```python
from build123d import *

# Parameters (mm, degrees)
SKETCH1_W                     = 46.5
SKETCH1_H                     = 83
BOSS_EXTRUDE1_DEPTH           = 7.540625
CUT_EXTRUDE3_START            = 7.540625
CUT_EXTRUDE3_DEPTH            = 2.38125
SKETCH10_R                    = 1.35255
CUT_EXTRUDE6_DEPTH            = 4.76885
SKETCH12_R                    = 3.175
BOSS_EXTRUDE2_DEPTH           = 5.159375
BOSS_EXTRUDE2_DRAFT           = 1
BOSS_EXTRUDE2_PROFILE_2_DEPTH = 5.159375
BOSS_EXTRUDE2_PROFILE_2_DRAFT = 1
BOSS_EXTRUDE2_PROFILE_3_DEPTH = 5.159375
BOSS_EXTRUDE2_PROFILE_3_DRAFT = 1
SKETCH12_R_2                  = 2.38125
BOSS_EXTRUDE2_PROFILE_4_DEPTH = 5.159375
BOSS_EXTRUDE2_PROFILE_4_DRAFT = 1
FILLET1_R                     = 3.175


with BuildPart() as part:
    # Sketch1 → Boss-Extrude1 (new body)
    with BuildSketch(Plane(origin=(0, 0, 0), x_dir=(1, 0, 0), z_dir=(0, 1, 0))):
        Rectangle(SKETCH1_W, SKETCH1_H)
    extrude(amount=BOSS_EXTRUDE1_DEPTH)

    # Sketch2 → Cut-Extrude3 (cut)
    with BuildSketch(Plane(origin=(0, 0, 0), x_dir=(1, 0, 0), z_dir=(0, 1, 0)).offset(CUT_EXTRUDE3_START)):
        with BuildLine():
            Line((5.926342072, -15.8450122), (16.691855897, 34.802748287))
            ThreePointArc((16.691855897, 34.802748287), (16.847821053, 35.78747353), (16.9, 36.783107142))
            Line((16.9, 36.783107142), (16.9, 41.5))
            Line((16.9, 41.5), (10.55, 41.5))
            Line((10.55, 41.5), (10.55, 36.783107142))
            ThreePointArc((10.55, 36.783107142), (10.532607018, 36.451229271), (10.480618632, 36.122987524))
            Line((10.480618632, 36.122987524), (4.2, 6.575))
            Line((4.2, 6.575), (1.742353127, 18.137319476))
            ThreePointArc((1.742353127, 18.137319476), (-7.787687338, 36.612083158), (-13.035, 16.49730565))
            Line((-13.035, 16.49730565), (-13.035, -10.23))
            ThreePointArc((-13.035, -10.23), (-11.164876798, -14.744876798), (-6.65, -16.615))
            Line((-6.65, -16.615), (3.2078125, -16.615))
            Line((3.2078125, -16.615), (3.2078125, -20.512873774))
            ThreePointArc((3.2078125, -20.512873774), (2.656919843, -22.538622657), (1.155983232, -24.006386448))
            ThreePointArc((1.155983232, -24.006386448), (0.870208506, -34.75413874), (10.438131483, -29.8499878))
            Line((10.438131483, -29.8499878), (14.4748, -29.8499878))
            ThreePointArc((14.4748, -29.8499878), (17.575454609, -28.565654609), (18.8597878, -25.465))
            Line((18.8597878, -25.465), (18.8597878, -20.23))
            ThreePointArc((18.8597878, -20.23), (17.575454609, -17.129345391), (14.4748, -15.8450122))
            Line((14.4748, -15.8450122), (5.926342072, -15.8450122))
        make_face()
        with BuildLine():
            Line((14.4748, -29.08), (10.43813073, -29.08))
            ThreePointArc((10.43813073, -29.08), (9.489135484, -26.135203334), (7.244016768, -24.006386448))
            ThreePointArc((7.244016768, -24.006386448), (5.743080157, -22.538622657), (5.1921875, -20.512873774))
            Line((5.1921875, -20.512873774), (5.1921875, -16.615))
            Line((5.1921875, -16.615), (14.4748, -16.615))
            ThreePointArc((14.4748, -16.615), (17.030991014, -17.673808986), (18.0898, -20.23))
            Line((18.0898, -20.23), (18.0898, -25.465))
            ThreePointArc((18.0898, -25.465), (17.030991014, -28.021191014), (14.4748, -29.08))
        make_face(mode=Mode.SUBTRACT)
        with BuildLine():
            Line((-4.021712531, 14.713303237), (2.473657928, -15.8450122))
            Line((2.473657928, -15.8450122), (-6.65, -15.8450122))
            ThreePointArc((-6.65, -15.8450122), (-10.620413203, -14.200413203), (-12.2650122, -10.23))
            Line((-12.2650122, -10.23), (-12.2650122, 15.993340762))
            ThreePointArc((-12.2650122, 15.993340762), (-8.267823292, 14.551807439), (-4.021712531, 14.713303237))
        make_face(mode=Mode.SUBTRACT)
    extrude(amount=-CUT_EXTRUDE3_DEPTH, mode=Mode.SUBTRACT)

    # Sketch10 → Cut-Extrude6 (cut)
    with BuildSketch(Plane(origin=(0, 7.540625, 0), x_dir=(1, 0, 0), z_dir=(0, 1, 0))):
        with Locations(Location((18.4747939, -22.8475, 0), (0, 0, 270))):
            Circle(SKETCH10_R)
        with Locations(Location((-12.6500061, 3.133652825, 0), (0, 0, 270))):
            Circle(SKETCH10_R)
    extrude(amount=-CUT_EXTRUDE6_DEPTH, mode=Mode.SUBTRACT)


with BuildPart() as boss_extrude2_tool:
    # Sketch12 → Boss-Extrude2 (with draft: the straight prism first)
    with BuildSketch(Plane(origin=(0, 7.540625, 0), x_dir=(1, 0, 0), z_dir=(0, 1, 0))):
        with Locations((-16.9, -35.15)):
            Circle(SKETCH12_R)
    extrude(amount=BOSS_EXTRUDE2_DEPTH)
    # Boss-Extrude2: the draft: its side faces are tilted about the plane it starts from
    boss_extrude2_sides = [boss_extrude2_tool.faces().sort_by_distance(p)[0] for p in [
        (-20.075, 10.1203125, 35.15),
    ]]
    draft(boss_extrude2_sides, Plane(origin=(0, 7.540625, 0), x_dir=(1, 0, 0), z_dir=(0, 1, 0)), BOSS_EXTRUDE2_DRAFT)


with BuildPart() as part_1:
    add(part.part)

    # Boss-Extrude2: add boss_extrude2_tool
    add(boss_extrude2_tool.part)


with BuildPart() as boss_extrude2_profile_2_tool:
    # Sketch12 → Boss-Extrude2 profile 2 (with draft: the straight prism first)
    with BuildSketch(Plane(origin=(0, 7.540625, 0), x_dir=(1, 0, 0), z_dir=(0, 1, 0))):
        with Locations((16.9, -35.15)):
            Circle(SKETCH12_R)
    extrude(amount=BOSS_EXTRUDE2_PROFILE_2_DEPTH)
    # Boss-Extrude2 profile 2: the draft: its side faces are tilted about the plane it starts from
    boss_extrude2_profile_2_sides = [boss_extrude2_profile_2_tool.faces().sort_by_distance(p)[0] for p in [
        (13.725, 10.1203125, 35.15),
    ]]
    draft(boss_extrude2_profile_2_sides, Plane(origin=(0, 7.540625, 0), x_dir=(1, 0, 0), z_dir=(0, 1, 0)), BOSS_EXTRUDE2_PROFILE_2_DRAFT)


with BuildPart() as part_2:
    add(part_1.part)

    # Boss-Extrude2 profile 2: add boss_extrude2_profile_2_tool
    add(boss_extrude2_profile_2_tool.part)


with BuildPart() as boss_extrude2_profile_3_tool:
    # Sketch12 → Boss-Extrude2 profile 3 (with draft: the straight prism first)
    with BuildSketch(Plane(origin=(0, 7.540625, 0), x_dir=(1, 0, 0), z_dir=(0, 1, 0))):
        with Locations((16.9, 9.75)):
            Circle(SKETCH12_R)
    extrude(amount=BOSS_EXTRUDE2_PROFILE_3_DEPTH)
    # Boss-Extrude2 profile 3: the draft: its side faces are tilted about the plane it starts from
    boss_extrude2_profile_3_sides = [boss_extrude2_profile_3_tool.faces().sort_by_distance(p)[0] for p in [
        (13.725, 10.1203125, -9.75),
    ]]
    draft(boss_extrude2_profile_3_sides, Plane(origin=(0, 7.540625, 0), x_dir=(1, 0, 0), z_dir=(0, 1, 0)), BOSS_EXTRUDE2_PROFILE_3_DRAFT)


with BuildPart() as part_3:
    add(part_2.part)

    # Boss-Extrude2 profile 3: add boss_extrude2_profile_3_tool
    add(boss_extrude2_profile_3_tool.part)


with BuildPart() as boss_extrude2_profile_4_tool:
    # Sketch12 → Boss-Extrude2 profile 4 (with draft: the straight prism first)
    with BuildSketch(Plane(origin=(0, 7.540625, 0), x_dir=(1, 0, 0), z_dir=(0, 1, 0))):
        with Locations((-18.4748, 36.7375)):
            Circle(SKETCH12_R_2)
    extrude(amount=BOSS_EXTRUDE2_PROFILE_4_DEPTH)
    # Boss-Extrude2 profile 4: the draft: its side faces are tilted about the plane it starts from
    boss_extrude2_profile_4_sides = [boss_extrude2_profile_4_tool.faces().sort_by_distance(p)[0] for p in [
        (-20.85605, 10.1203125, -36.7375),
    ]]
    draft(boss_extrude2_profile_4_sides, Plane(origin=(0, 7.540625, 0), x_dir=(1, 0, 0), z_dir=(0, 1, 0)), BOSS_EXTRUDE2_PROFILE_4_DRAFT)


with BuildPart() as part_4:
    add(part_3.part)

    # Boss-Extrude2 profile 4: add boss_extrude2_profile_4_tool
    add(boss_extrude2_profile_4_tool.part)

    # Fillet1
    fillet1_edges = [part_4.edges().sort_by_distance(p)[0] for p in [
        (23.25, 3.7703125, 41.5),
        (-23.25, 3.7703125, 41.5),
        (-23.25, 3.7703125, -41.5),
    ]]
    fillet(fillet1_edges, radius=FILLET1_R)


solid = part_4.part
```
Input: part model. Units: mm. Frame: model coordinates. A direction names the side the tool comes from. Give positions to 0.01 mm unless a question says otherwise; leave off trailing zeros. Order: outer loops, then holes, each group sorted by start corner. A loop starts at its lowest first (then second) coordinate and runs counter-clockwise, first axis right, second up.
1. Section A-A on y = 6.75. Give the number of separate pieces and of enclosed holes in the cut face, and give its area (3 significant figures).
Derived:
separate pieces: 3
enclosed holes: 0
area: 2,790 mm2
2. Mould query, pull axis X, two halves, no side actions, for faces 1 (the flat face through (-2, 6, 16.615)), 2 (the flat face through (23.25, 4, -1)), 3 (the flat face through (17, 12.7, -10)). Classes: released by +X, released by -X, zero draft, split by the parting line, or undercut.
Derived:
face 1: undercut
face 2: released by +X
face 3: zero draft
3. Section B-B on z = -25.55. Return the cut outline in (x, y), and give its area (3 significant figures).
Derived:
outline: (-23.25, 0) - (23.25, 0) - (23.25, 7.54) - (14.73, 7.54) - (14.73, 5.16) - (8.23, 5.16) - (8.23, 7.54) - (4.57, 7.54) - (4.57, 5.16) - (-17.69, 5.16) - (-17.69, 7.54) - (-23.25, 7.54) - close
area: 282 mm2
4. Pin query (flat end, axial travel): pin 1 (4.5 mm diameter, centred on x = -8, z = -6, fed in from +Y); pin 2 (5 mm diameter, centred on y = 10.5, z = -23.5, fed in from -X); pin 3 (10 mm diameter, centred on x = -14, z = 30.5, fed in from +Y); pin 4 (20 mm diameter, centred on x = -6.56, z = -25.55, fed in from +Y). Return the tip coordinate at first contact, or that it passes through.
Derived:
pin 1: stops at y = 7.54
pin 2: passes through
pin 3: stops at y = 12.7
pin 4: stops at y = 5.16
5. Reachability of faces 4 (the flat face through (16.9, 6, -39)), 5 (the flat face through (-0.82, 6.37, 0.35)), 6 (the flat face through (0, 0, -1)) from +Z, -Z, +X, -X, +Y, -Y: full face, straight path, thin tool, end or side. Return the list, or none.
Derived:
face 4: -Z, +Y
face 5: +Y
face 6: +Z, -Z, +X, -X, -Y
6. Material intervals for L1, parallel to Z at x = -6, y = 7 (3 decimals); L2, parallel to X at y = 5.25, z = -6 (3 decimals); L3, parallel to Y at x = -0.5, z = 8, sorted ascending.
Derived:
L1: z = -41.5 to -36.666, -14.434 to 15.845, 16.615 to 41.5
L2: x = -23.25 to -13.035, -12.265 to -2.17, 10.57 to 23.25
L3: y = 0 to 7.54
